from build123d import *

# Parameters (mm, degrees)
SKETCH1_R           = 2.5
BOSS_EXTRUDE3_DEPTH = 13.5
SKETCH2_R           = 14
BOSS_EXTRUDE4_DEPTH = 0.25
CHAMFER1_SIZE       = 0.25


with BuildPart() as part:
    # Sketch1 → Boss-Extrude3 (new, symmetric)
    with BuildSketch(Plane(origin=(0, 0, 0), x_dir=(0, 0, -1), z_dir=(1, 0, 0))):
        Circle(SKETCH1_R)
    extrude(amount=BOSS_EXTRUDE3_DEPTH, both=True)

    # Sketch2 → Boss-Extrude4 (add, symmetric)
    with BuildSketch(Plane(origin=(0, 0, 0), x_dir=(0, 0, -1), z_dir=(1, 0, 0))):
        Circle(SKETCH2_R)
    extrude(amount=BOSS_EXTRUDE4_DEPTH, both=True)

    # Chamfer1
    chamfer1_edges = [part.edges().sort_by_distance(p)[0] for p in [
        (-0.25, 0, 14),
        (0.25, 0, 14),
    ]]
    chamfer(chamfer1_edges, length=CHAMFER1_SIZE - 0.0001)  # a hair under: the kernel refuses the full size


solid = part.part
Model file for the job. Use its own axes, mm. A direction names the side the tool comes from. Coordinates: 2 decimals unless noted, no trailing zeros. Order: outer loops, then holes, each group sorted by start corner. A loop starts at its lowest first (then second) coordinate and runs counter-clockwise, first axis right, second up. Notation, with made-up numbers: (87.5, 84.5) -> (140.5, 84.5) arc R37 ccw to (140.5, 121.5) -> close; hole circle Ø2 at (83.5, -24). An arc over 180 degrees is marked (long way). Return JSON: item names as keys, results as strings. Group by question number.
Item 1: Wall check: line 1 along X through (y, z) = (-12.5, -3.25); line 2 along Y through (x, z) = (-12, 2). Give the ranges that are in metal, low to high. Write a range as [from, to].
Item 2: Tool access for faces 1 (the cylindrical face through (6.97, -2.44, 0.54)), 2 (the flat face through (13.5, 0, 0)), 3 (the cylindrical face through (-6.78, -2.44, 0.54)): list every direction of +Z, -Z, +X, -X, +Y, -Y with a clear straight run to the whole face (end or side of a thin tool).
Item 3: Saw through at C-C on x = 1. Write the cut outline in (y, z).
Item 4: Flat gauge pins, fed straight in: P1, Ø1.5, axis at y = 0, z = 7.5, coming from the +X side; P2, Ø5, axis at x = -0.5, y = 4.5, coming from the -Z side; P3, Ø4, axis at x = -2.5, y = -2, coming from the -Z side. Where does each tip first touch, or does it go through?
Values found:
{
 "1": {"line 1": "x = [-0.25, 0.25]", "line 2": "y = [-1.5, 1.5]"},
 "2": {"face 1": "+X", "face 2": "+Z, -Z, +X, +Y, -Y", "face 3": "-X"},
 "3": {"outline": "circle Ø5 at (0, 0)"},
 "4": {"P1": "stops at x = 0.25", "P2": "stops at z = -13.85", "P3": "stops at z = -2.5"}
}
